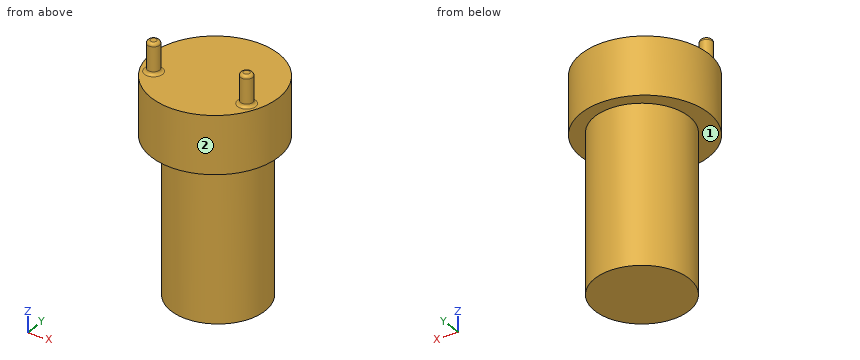
```python
from build123d import *

# Parameters (mm, degrees)
SKETCH1_R           = 15.5
BOSS_EXTRUDE1_DEPTH = 52
SKETCH2_R           = 21
BOSS_EXTRUDE2_DEPTH = 19
SKETCH3_R           = 2
BOSS_EXTRUDE3_DEPTH = 10
FILLET1_R           = 1


with BuildPart() as part:
    # Sketch1 → Boss-Extrude1 (new body)
    with BuildSketch(Plane.XY):
        with Locations(Location((0, 0, 0), (0, 0, 180))):
            Circle(SKETCH1_R)
    extrude(amount=BOSS_EXTRUDE1_DEPTH)

    # Sketch2 → Boss-Extrude2 (add)
    with BuildSketch(Plane.XY.offset(52)):
        with Locations((0, -1.5)):
            Circle(SKETCH2_R)
    extrude(amount=BOSS_EXTRUDE2_DEPTH)

    # Sketch3 → Boss-Extrude3 (add)
    with BuildSketch(Plane.XY.offset(71)):
        with Locations((-15.337121903, -8.854891459)):
            Circle(SKETCH3_R)
        with Locations(Location((15.337121903, -8.854891459, 0), (0, 0, 180))):
            Circle(SKETCH3_R)
    extrude(amount=BOSS_EXTRUDE3_DEPTH)

    # Fillet1
    fillet1_edges = [part.edges().sort_by_distance(p)[0] for p in [
        (-17.337121903, -8.854891459, 71),
        (-17.337121903, -8.854891459, 81),
        (17.337121903, -8.854891459, 71),
        (17.337121903, -8.854891459, 81),
    ]]
    fillet(fillet1_edges, radius=FILLET1_R)


solid = part.part
```
The listing builds one solid part. Answer for the finished solid, in the listing's coordinates (mm). Face numbers are marked on the shaded views. A direction names the side the tool comes from. Give positions to 0.01 mm unless a question says otherwise; leave off trailing zeros. Loops run counter-clockwise (first coordinate to the right, second up) from the corner with the lowest first, then second, coordinate; pieces in that order, holes last. Notation, with made-up numbers: M 85.5,26.5 L 95.5,26.5 A8 cw 95.5,37.5 Z; hole C -26,28 d4. An arc over 180 degrees is marked long. One line per item, written item: value.
1. Section A-A on x = 0 is taken. Determine the outline of the cut face in (y, z), plus the area to 3 significant figures.
Found:
outline: M -22.5,52 L -15.5,52 L -15.5,0 L 15.5,0 L 15.5,52 L 19.5,52 L 19.5,71 L -22.5,71 Z
area: 2,410 mm^2
2. Section B-B on y = 1 is taken. Determine the outline of the cut face in (x, z), plus the area to 3 significant figures.
Found:
outline: M -20.85,52 L -15.47,52 L -15.47,0 L 15.47,0 L 15.47,52 L 20.85,52 L 20.85,71 L -20.85,71 Z
area: 2,400 mm^2
3. Each of these flat-tipped pins is pushed along its axis until it touches: P1, Ø4, axis at y = -8.5, z = 55.5, coming from the +X side; P2, Ø1, axis at x = -9, z = 21, coming from the +Y side; P3, Ø21, axis at x = 0, y = -8.5, coming from the +Z side. Where does it stop, or does it pass through?
Found:
P1: x = 20.4
P2: y = 12.96
P3: z = 71
4. Section C-C on z = 42 is taken. Determine the outline of the cut face in (x, y), plus the area to 3 significant figures.
Found:
outline: C 0,0 d31
area: 755 mm^2
5. Find the intervals of material crossed by probe 1 along Z at (x, y) = (15, 11); probe 2 along Z at (x, y) = (7, -3); probe 3 along Y at (x, z) = (6, 66), in increasing order.
Found:
probe 1: 52 to 71
probe 2: 0 to 71
probe 3: -21.62 to 18.62
6. For the marked faces 1 and 2, determine the directions among +Z, -Z, +X, -X, +Y, -Y from which every point of the face is accessible in a straight line to the end or side of a thin tool.
Found:
face 1: -Z
face 2: +Z, -Z
